Geometry: final body of the model. Coordinates: model frame, mm. A direction names the side the tool comes from. Give positions to 0.01 mm unless a question says otherwise; leave off trailing zeros. Write each loop counter-clockwise with the first axis right and the second up, starting at its lowest first coordinate (ties: lowest second). Pieces come first, ordered by that corner, then holes. Notation, with made-up numbers: (39, 52.5) -> (73, 52.5) arc R19 cw to (73, 58.5) -> close; hole circle Ø7 at (70.5, 40). An arc over 180 degrees is marked (long way). Answer in a Markdown table with one row per item. Add a question column.
Item 1: Section query A-A on y = -11.5. Output: boundary loops of the cut face in (x, z).
Item 2: First-contact query: P1, Ø4, axis at x = -0.5, y = 14, coming from the +Z side; P2, Ø4, axis at x = -15.5, z = 30, coming from the +Y side; P3, Ø12, axis at x = 1, z = 17, coming from the -Y side. Flat tips, straight axial feed; report the tip coordinate or a pass-through.
Item 3: Section query B-B on z = 35. Output: boundary loops of the cut face in (x, y).
Item 4: Section query C-C on y = 14. Output: boundary loops of the cut face in (x, z).
Item 5: Draft query along X for faces 5 (the flat face through (25, 0, 2)), 6 (the flat face through (0, 0, 55)), 7 (the cylindrical face through (-2, 13.5, 6.5)). Return one class per face: +X half, -X half, draft (parallel to the pull), parting line (faces both ways), or undercut.
Item 6: Access query for faces 1 (the flat face through (0, -25, 2)), 2 (the flat face through (15, 0, 8)), 3 (the cylindrical face through (17.384, 0.753, 6.479)), 4 (the flat face through (0, -15, 8)). Directions: +Z, -Z, +X, -X, +Y, -Y. A direction counts if a zero-diameter tool reaches every point of the face in a straight line with its end or side. Return the directions, or none.
Item 7: Material intervals for probe 1 along Z at (x, y) = (14, 19); probe 2 along Y at (x, z) = (-22.5, 20.5); probe 3 along Y at (x, z) = (19.5, 35), sorted ascending. Write a range as from..to.
Solid Edge part; units mm, degrees
sketch "Sketch1" plane through (0, 0, 0) normal (0, 0, 1) x (1, 0, 0)
  line L0 (-25, -25) -> (25, -25)
  line L1 (25, -25) -> (25, 25)
  line L2 (25, 25) -> (-25, 25)
  line L3 (-25, 25) -> (-25, -25)
extrude "Protrusion1" add sketch "Sketch1" along normal blind 5
sketch "Sketch2" plane through (0, 0, 5) normal (0, 0, 1) x (0, -1, 0)
  line L0 (25, 24) -> (1, 0)
  line L1 (1, 0) -> (25, -24)
  line L2 (24, -25) -> (25, -24)
  line L3 (24, -25) -> (0, -1)
  line L4 (0, -1) -> (-24, -25)
  line L5 (-24, -25) -> (-25, -24)
  line L6 (-25, -24) -> (-1, 0)
  line L7 (-25, 24) -> (-1, 0)
  line L8 (-25, 24) -> (-24, 25)
  line L9 (-24, 25) -> (0, 1)
  line L10 (0, 1) -> (24, 25)
  line L11 (24, 25) -> (25, 24)
extrude "Kihúzás_2" add sketch "Sketch2" along normal blind 50
sketch "Sketch3" plane through (0, 13, 5) normal (0, 0, 1) x (0.7071, -0.7071, 0)
  circle A0 centre (-1.4142, 1.4142) radius 2.5
  circle A1 centre (19.799, 1.4142) radius 2.5
  circle A2 centre (19.799, -19.799) radius 2.5
  circle A3 centre (-1.4142, -19.799) radius 2.5
extrude "Kihúzás_3" add sketch "Sketch3" along normal blind 3
Findings below:
| question | item | result |
|---|---|---|
| 1 | outline | (-25, 0) -> (25, 0) -> (25, 5) -> (12.5, 5) -> (12.5, 55) -> (10.5, 55) -> (10.5, 5) -> (-10.5, 5) -> (-10.5, 55) -> (-12.5, 55) -> (-12.5, 5) -> (-25, 5) -> close |
| 2 | P1 | stops at z = 8 |
| 2 | P2 | stops at y = 18.5 |
| 2 | P3 | stops at y = -8 |
| 3 | outline | (-25, -24) -> (-24, -25) -> (0, -1) -> (24, -25) -> (25, -24) -> (1, 0) -> (25, 24) -> (24, 25) -> (0, 1) -> (-24, 25) -> (-25, 24) -> (-1, 0) -> close |
| 4 | outline | (-25, 0) -> (25, 0) -> (25, 5) -> (15, 5) -> (15, 55) -> (13, 55) -> (13, 5) -> (2.29, 5) -> (2.29, 8) -> (-2.29, 8) -> (-2.29, 5) -> (-13, 5) -> (-13, 55) -> (-15, 55) -> (-15, 5) -> (-25, 5) -> close |
| 5 | face 5 | +X half |
| 5 | face 6 | draft |
| 5 | face 7 | undercut |
| 6 | face 1 | +Z, -Z, +X, -X, -Y |
| 6 | face 2 | +Z, +X |
| 6 | face 3 | +Z |
| 6 | face 4 | +Z, -Y |
| 7 | probe 1 | z = 0..5 |
| 7 | probe 2 | y = -23.5..-21.5, 21.5..23.5 |
| 7 | probe 3 | y = -20.5..-18.5, 18.5..20.5 |
